```python
from build123d import *

# Parameters (mm, degrees)
CROQUIS1_W              = 36
CROQUIS1_H              = 7
CROQUIS1_R              = 2.6
SALIENTE_EXTRUIR1_DEPTH = 10
CORTAR_EXTRUIR1_DEPTH   = 7
CROQUIS4_W              = 11.4
CROQUIS4_H              = 10
SALIENTE_EXTRUIR2_DEPTH = 5
REDONDEO1_R             = 2


with BuildPart() as part:
    # Croquis1 → Saliente-Extruir1 (new body)
    with BuildSketch(Plane.XY):
        with Locations((-28.016694491, 12.37804878)):
            Rectangle(CROQUIS1_W, CROQUIS1_H)
        with Locations((-42.516694491, 12.37804878)):
            Circle(CROQUIS1_R, mode=Mode.SUBTRACT)
        with Locations((-13.516694491, 12.37804878)):
            Circle(CROQUIS1_R, mode=Mode.SUBTRACT)
    extrude(amount=SALIENTE_EXTRUIR1_DEPTH)

    # Croquis2 → Cortar-Extruir1 (cut)
    with BuildSketch(Plane.XZ.offset(-8.87804878)):
        Polygon((-29.816694491, 5), (-32.166694491, 9.070319398), (-36.866694491, 9.070319398), (-39.216694491, 5), (-36.866694491, 0.929680602), (-32.166694491, 0.929680602), align=None)
    extrude(amount=-CORTAR_EXTRUIR1_DEPTH, mode=Mode.SUBTRACT)

    # Croquis4 → Saliente-Extruir2 (add)
    with BuildSketch(Plane.XZ.offset(-8.87804878)):
        with Locations((-34.516694491, 5)):
            Rectangle(CROQUIS4_W, CROQUIS4_H)
        Polygon((-29.816694491, 5), (-32.166694491, 9.070319398), (-36.866694491, 9.070319398), (-39.216694491, 5), (-36.866694491, 0.929680602), (-32.166694491, 0.929680602), align=None, mode=Mode.SUBTRACT)
    extrude(amount=SALIENTE_EXTRUIR2_DEPTH)

    # Redondeo1
    redondeo1_edges = [part.edges().sort_by_distance(p)[0] for p in [
        (-10.016694491, 15.87804878, 5),
        (-10.016694491, 8.87804878, 5),
        (-46.016694491, 8.87804878, 5),
        (-46.016694491, 15.87804878, 5),
    ]]
    fillet(redondeo1_edges, radius=REDONDEO1_R)


solid = part.part
```
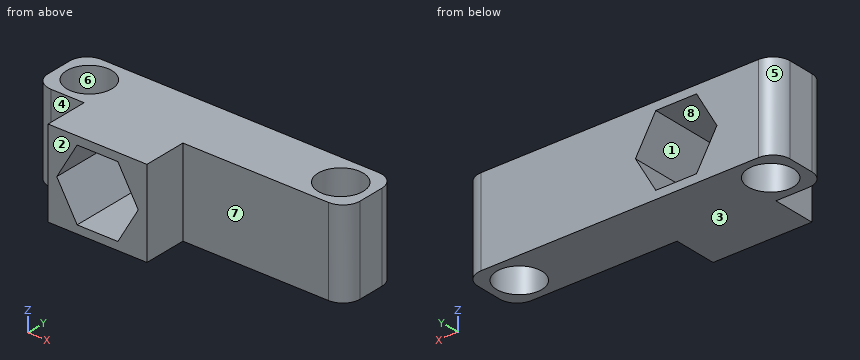
The model under review builds one solid part; all positions refer to its coordinate system, in mm. Face numbers are marked on the shaded views. A direction names the side the tool comes from. Round coordinates to 2 decimals unless told otherwise and drop trailing zeros. Loops run counter-clockwise (first coordinate to the right, second up) from the corner with the lowest first, then second, coordinate; pieces in that order, holes last. Notation, with made-up numbers: M 7.25,72 L 55.25,72 A29 ccw 55.25,98 Z; hole C 50,53.5 d10. An arc over 180 degrees is marked long. Answer as a JSON object with one key per item and string values.
(1) Tool access review of the marked faces 4, 5, 6, 7 and 8: name each direction out of +Z, -Z, +X, -X, +Y, -Y from which nothing blocks a thin tool from reaching the whole face with its end or side.
Resolved:
{"face 4": "+Z, -Z, -X, -Y", "face 5": "+Z, -Z, -X, +Y", "face 6": "+Z, -Z", "face 7": "+Z, -Z, +X, -Y", "face 8": "+Y, -Y"}
(2) Draft analysis for pull direction Z (two halves, no side actions). For the marked faces 1, 2 and 3, state which applies: released by +Z, released by -Z, zero draft, split by the parting line, or undercut.
Resolved:
{"face 1": "undercut", "face 2": "zero draft", "face 3": "released by -Z"}
(3) Clearance check with flat-ended pins moving along their axes: P1, Ø3, axis at x = -43, z = 6, coming from the -Y side; P2, Ø1.5, axis at y = 6, z = 6.5, coming from the +X side; P3, Ø4, axis at y = 6, z = 3, coming from the -X side. State where each tip first meets the part, or that it passes through.
Resolved:
{"P1": "y = 8.88", "P2": "x = -28.82", "P3": "x = -40.22"}
(4) Take a section at C-C on y = 5.75. Give the boundary of the cut face in (x, z).
Resolved:
{"outline": "M -40.22,0 L -28.82,0 L -28.82,10 L -40.22,10 Z; hole M -39.22,5 L -36.87,0.93 L -32.17,0.93 L -29.82,5 L -32.17,9.07 L -36.87,9.07 Z"}
(5) Take a section at B-B on x = -35. Give the boundary of the cut face in (y, z), and give its area (3 significant figures).
Resolved:
{"outline": "M 3.88,0 L 15.88,0 L 15.88,0.93 L 3.88,0.93 Z; M 3.88,9.07 L 15.88,9.07 L 15.88,10 L 3.88,10 Z", "area": "22.3 mm²"}
(6) To check wall thickness, follow line 1 along Y through (x, z) = (-13.5, 0.75); line 2 along Z through (x, y) = (-35, 5); line 3 along X through (y, z) = (11.5, 0.75). State the ranges of each line that lie inside material, in increasing order.
Resolved:
{"line 1": "8.88 to 9.78, 14.98 to 15.88", "line 2": "0 to 0.93, 9.07 to 10", "line 3": "-46.02 to -44.96, -40.07 to -15.96, -11.07 to -10.02"}
(7) Take a section at A-A on z = 8. Give the boundary of the cut face in (x, y), and give its area (3 significant figures).
Resolved:
{"outline": "M -46.02,10.88 A2 ccw -44.02,8.88 L -40.22,8.88 L -40.22,3.88 L -37.48,3.88 L -37.48,15.88 L -44.02,15.88 A2 ccw -46.02,13.88 Z; M -31.55,3.88 L -28.82,3.88 L -28.82,8.88 L -12.02,8.88 A2 ccw -10.02,10.88 L -10.02,13.88 A2 ccw -12.02,15.88 L -31.55,15.88 Z; hole C -42.52,12.38 d5.2; hole C -13.52,12.38 d5.2", "area": "192 mm²"}
(8) Take a section at D-D on y = 14.5. Give the boundary of the cut face in (x, z).
Resolved:
{"outline": "M -45.92,0 L -44.02,0 L -44.02,10 L -45.92,10 Z; M -41.01,0 L -15.02,0 L -15.02,10 L -41.01,10 Z; M -12.01,0 L -10.12,0 L -10.12,10 L -12.01,10 Z; hole M -39.22,5 L -36.87,0.93 L -32.17,0.93 L -29.82,5 L -32.17,9.07 L -36.87,9.07 Z"}
